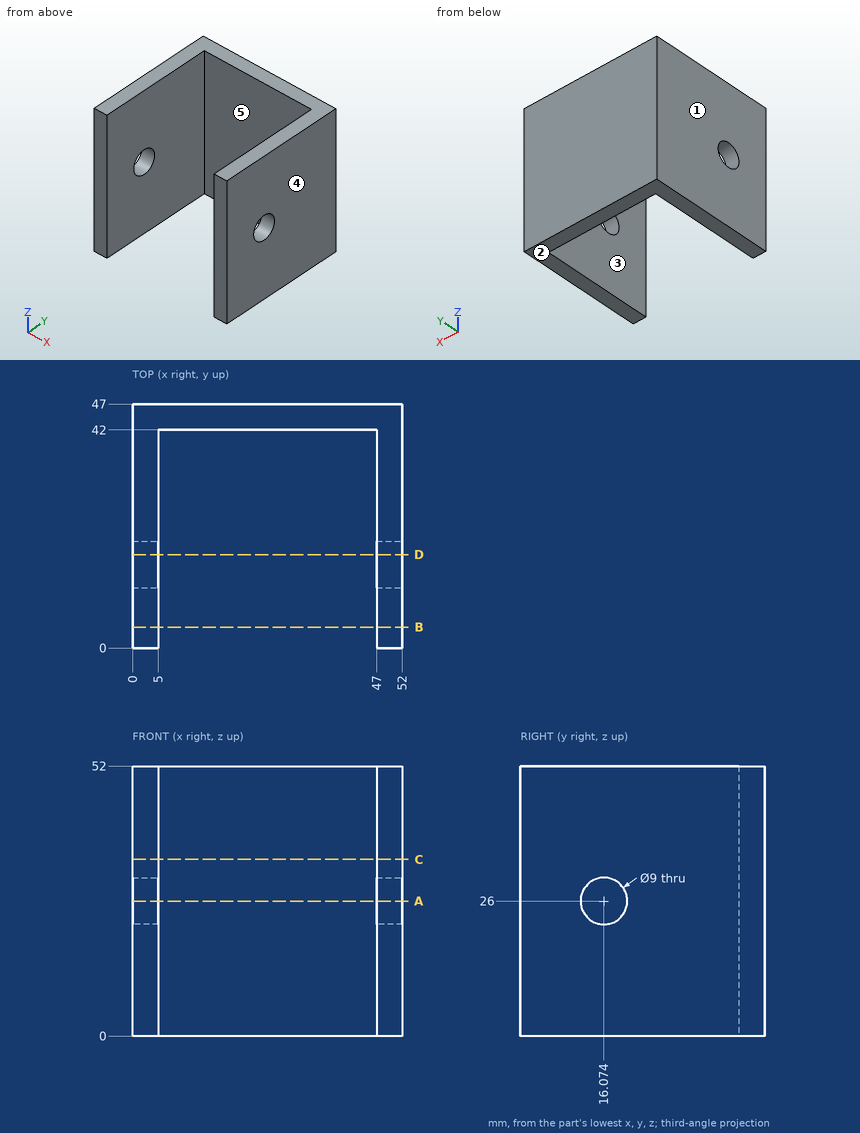
Job drawing, mm, ordinate dimensions from the low corner. One solid piece. A direction names the side the tool comes from. Give positions to 0.01 mm unless a question says otherwise; leave off trailing zeros. Write each loop counter-clockwise with the first axis right and the second up, starting at its lowest first coordinate (ties: lowest second). Pieces come first, ordered by that corner, then holes. Notation, with made-up numbers: (-16.75, -23) -> (20.25, -23) arc R29 cw to (20.25, 3) -> close; hole circle Ø11 at (20, -35). An arc over 180 degrees is marked (long way). Return JSON: item names as keys, results as strings.
Item 1: Two-plate mould, pull along X, no slides. Class the marked faces 1, 2 and 3: +X half, -X half, draft (parallel to the pull), parting line (faces both ways), or undercut.
Answer below:
{"face 1": "-X half", "face 2": "draft", "face 3": "undercut"}
Item 2: Band-saw the part on C-C (z = 34). List the corners of the cut face in (x, y).
Answer below:
{"outline": "(0, 0) -> (5, 0) -> (5, 42) -> (47, 42) -> (47, 0) -> (52, 0) -> (52, 47) -> (0, 47) -> close"}
Item 3: Band-saw the part on A-A (z = 26). List the corners of the cut face in (x, y).
Answer below:
{"outline": "(0, 0) -> (5, 0) -> (5, 11.57) -> (0, 11.57) -> close; (0, 20.57) -> (5, 20.57) -> (5, 42) -> (47, 42) -> (47, 20.57) -> (52, 20.57) -> (52, 47) -> (0, 47) -> close; (47, 0) -> (52, 0) -> (52, 11.57) -> (47, 11.57) -> close"}
Item 4: Tool access for the marked faces 4 and 5: list every direction of +Z, -Z, +X, -X, +Y, -Y with a clear straight run to the whole face (end or side of a thin tool).
Answer below:
{"face 4": "+Z, -Z, +X, +Y, -Y", "face 5": "+Z, -Z, -Y"}
Item 5: Band-saw the part on D-D (y = 18). List the corners of the cut face in (x, z), then the cut area to 3 significant figures.
Answer below:
{"outline": "(0, 0) -> (5, 0) -> (5, 21.93) -> (0, 21.93) -> close; (0, 30.07) -> (5, 30.07) -> (5, 52) -> (0, 52) -> close; (47, 0) -> (52, 0) -> (52, 21.93) -> (47, 21.93) -> close; (47, 30.07) -> (52, 30.07) -> (52, 52) -> (47, 52) -> close", "area": "439 mm2"}
Item 6: Drill centre lines: probe 1 along Y at (x, z) = (3, 26); probe 2 along X at (y, z) = (40.5, 6); probe 3 along Y at (x, z) = (21.5, 34). Where is each one in solid material? Low to high.
Answer below:
{"probe 1": "y = 0 to 11.57, 20.57 to 47", "probe 2": "x = 0 to 5, 47 to 52", "probe 3": "y = 42 to 47"}
Item 7: Drop flat-ended pins along their axis: pin 1 (10.5 mm diameter, centred on y = 16.074, z = 26, fed in from -X); pin 2 (8 mm diameter, centred on x = 18, z = 33.5, fed in from -Y); pin 3 (8 mm diameter, centred on y = 16.074, z = 26, fed in from -X). Give the stop position or say it passes through.
Answer below:
{"pin 1": "stops at x = 0", "pin 2": "stops at y = 42", "pin 3": "passes through"}
Item 8: Band-saw the part on B-B (y = 4). List the corners of the cut face in (x, z), then the cut area to 3 significant figures.
Answer below:
{"outline": "(0, 0) -> (5, 0) -> (5, 52) -> (0, 52) -> close; (47, 0) -> (52, 0) -> (52, 52) -> (47, 52) -> close", "area": "520 mm2"}
